```python
from build123d import *

# Parameters (mm, degrees)
F0_R     = 19.05
F0_R_2   = 9.525
F1_DEPTH = 0.303999
F0_R_3   = 7.1501
F2_DEPTH = 0.553999
F3_DEPTH = 1.303999


with BuildPart() as f1:
    # F0 (on Top) → F1 (new body)
    with BuildSketch(Plane.XY):
        Circle(F0_R)
        Circle(F0_R_2, mode=Mode.SUBTRACT)
    extrude(amount=F1_DEPTH)

    # F0 (on Top) → F2 (join)
    with BuildSketch(Plane.XY):
        Circle(F0_R_2)
        Circle(F0_R_3, mode=Mode.SUBTRACT)
    extrude(amount=F2_DEPTH)

    # F0 (on Top) → F3 (join)
    with BuildSketch(Plane.XY):
        Circle(F0_R_3)
    extrude(amount=F3_DEPTH)


solid = f1.part
```
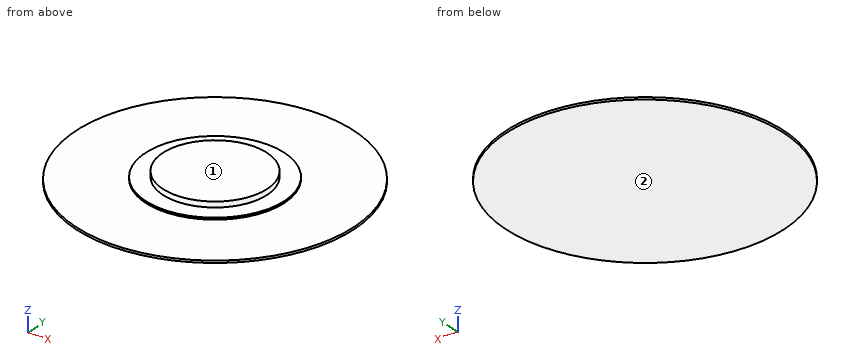
Can you work these out from the model? Positions are in its coordinate system, mm. Face numbers are marked on the shaded views. Round coordinates to 2 decimals unless told otherwise and drop trailing zeros. Loops run counter-clockwise (first coordinate to the right, second up) from the corner with the lowest first, then second, coordinate; pieces in that order, holes last. Notation, with made-up numbers: (-25, 52) -> (12, 52) arc R37 cw to (12, 88) -> close; hole circle Ø5 at (-21.75, -13). An arc over 180 degrees is marked (long way). One line per item, written item: value. Start each with the question number.
1. If we mould it in two halves opening along Z, with no side actions, what happens to the marked faces 1 and 2? For each: pulls with the +Z half, pulls with the -Z half, needs draft (parallel to the pull), parting line crosses it, or undercut.
2. If we section it at A-A, the plane x = -3.5: Write out the boundary of the cut face in (y, z).
3. If we section it at B-B, the plane y = 0: Write out the boundary of the cut face in (x, z) (3 decimals), then the cut area to 3 significant figures.
4. If I drill on probe 1 along Z at (x, y) = (9.5, -3.5); probe 2 along Z at (x, y) = (6, -4); probe 3 along X at (y, z) = (2.5, 0.35), over which ranges is the centre line in solid material (lowest first)?
5. If we section it at C-C, the plane z = 0.8: Write out the boundary of the cut face in (x, y).
6. If we section it at D-D, the plane x = 8: Write out the boundary of the cut face in (y, z), then the cut area to 3 significant figures.
7. For pin 1 (10 mm diameter, centred on x = -1.5, y = 13.5, fed in from +Z), with a flat end and sliding along its axis, tell me the tip position at first contact or that it passes through.
Calculated:
1. face 1: pulls with the +Z half
1. face 2: pulls with the -Z half
2. outline: (-18.73, 0) -> (18.73, 0) -> (18.73, 0.3) -> (8.86, 0.3) -> (8.86, 0.55) -> (6.23, 0.55) -> (6.23, 1.3) -> (-6.23, 1.3) -> (-6.23, 0.55) -> (-8.86, 0.55) -> (-8.86, 0.3) -> (-18.73, 0.3) -> close
3. outline: (-19.05, 0) -> (19.05, 0) -> (19.05, 0.304) -> (9.525, 0.304) -> (9.525, 0.554) -> (7.15, 0.554) -> (7.15, 1.304) -> (-7.15, 1.304) -> (-7.15, 0.554) -> (-9.525, 0.554) -> (-9.525, 0.304) -> (-19.05, 0.304) -> close
3. area: 27.1 mm²
4. probe 1: z = 0 to 0.3
4. probe 2: z = 0 to 0.55
4. probe 3: x = -9.19 to 9.19
5. outline: circle Ø14.3 at (0, 0)
6. outline: (-17.29, 0) -> (17.29, 0) -> (17.29, 0.3) -> (5.17, 0.3) -> (5.17, 0.55) -> (-5.17, 0.55) -> (-5.17, 0.3) -> (-17.29, 0.3) -> close
6. area: 13.1 mm²
7. pin 1: stops at z = 0.55
